Geometry: see drawing. Coordinates: mm, zero at the bounding-box minimum. A direction names the side the tool comes from. Coordinates: 2 decimals unless noted, no trailing zeros. Loops run counter-clockwise (first coordinate to the right, second up) from the corner with the lowest first, then second, coordinate; pieces in that order, holes last. Notation, with made-up numbers: (47, 72) -> (103, 72) arc R14 ccw to (103, 87) -> close; hole circle Ø9 at (-39.5, -40). An arc over 180 degrees is marked (long way). One line per item, written item: value. Start each with the question number.
Item 1: Contact query for a flat-ended pin moving along its axis: pin 1 Ø6 at (x, z) = (22, 27.5) entering from +Y. Output: stop coordinate, or through.
Item 2: Section query B-B on z = 5. Return loops of the section in (x, y).
Item 3: Mould query, pull axis Y, two halves, no side actions, for the marked faces 3, 4, 5 and 6. Classes: +Y half, -Y half, draft (parallel to the pull), parting line (faces both ways), or undercut.
Item 4: Ray query, probe 1 along Y at (x, z) = (24, 32); probe 2 along Y at (x, z) = (24.5, 16); probe 3 along Y at (x, z) = (18.75, 5). Return the intervals inside material, ascending. Write a range as from..to.
Item 5: Set-up query: the marked faces 1 and 2. Return all of +Z, -Z, +X, -X, +Y, -Y with unobstructed straight access to the full face (end or side cutting, diameter ignored); none if empty.
Item 6: Section query D-D on y = 33. Return loops of the section in (x, z), then the cut area to 3 significant figures.
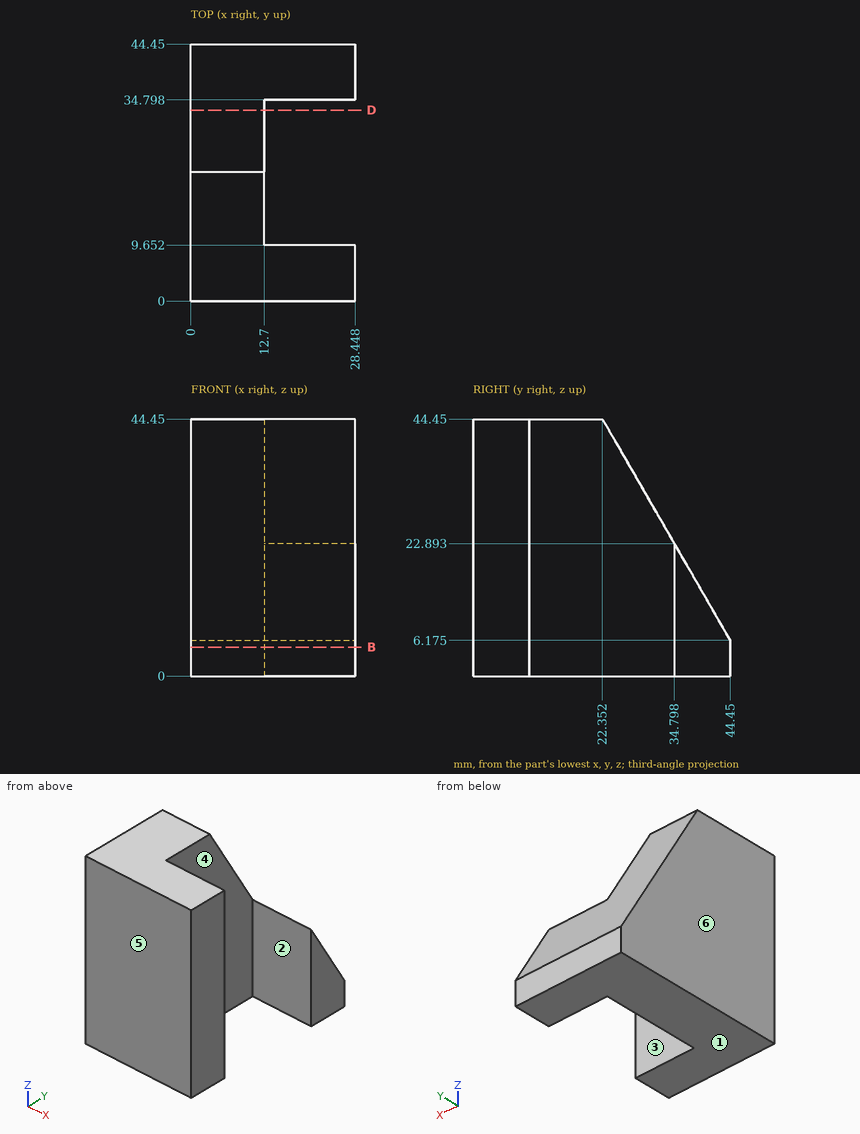
Reply:
1. pin 1: stops at y = 9.65
2. outline: (0, 0) -> (28.45, 0) -> (28.45, 9.65) -> (12.7, 9.65) -> (12.7, 34.8) -> (28.45, 34.8) -> (28.45, 44.45) -> (0, 44.45) -> close
3. face 3: undercut
3. face 4: undercut
3. face 5: -Y half
3. face 6: draft
4. probe 1: y = 0..9.65
4. probe 2: y = 0..9.65, 34.8..38.78
4. probe 3: y = 0..9.65, 34.8..44.45
5. face 1: -Z, +X, -X, +Y, -Y
5. face 2: +Z, -Z, +X
6. outline: (0, 0) -> (12.7, 0) -> (12.7, 26.01) -> (0, 26.01) -> close
6. area: 330 mm²
